from build123d import *

# Parameters (mm, degrees)
BOSS_EXTRUDE2_DEPTH = 16
CUT_EXTRUDE2_DEPTH  = 1
SKETCH6_R           = 0.8
CUT_EXTRUDE4_DEPTH  = 20


with BuildPart() as part:
    # Sketch1 → Revolve2 (revolve)
    with BuildSketch(Plane.XY, mode=Mode.PRIVATE) as revolve2_sk:
        with BuildLine():
            Line((8.97393545, 70), (10, 70))
            Line((10, 70), (10, 85))
            Line((10, 85), (5, 85))
            Line((5, 85), (5, 81.038856971))
            Line((5, 81.038856971), (-25, 81.038856971))
            Line((-25, 81.038856971), (-25, 85))
            Line((-25, 85), (-30, 85))
            Line((-30, 85), (-30, 70))
            add(Edge.make_bspline(
                [(-30, 70), (-18.635717154, 58.062094), (-15, 10)],
                knots=[0, 0, 0, 1, 1, 1], degree=2, weights=[1, 2.302666222, 1]))
            Line((-15, 10), (-15, 0))
            Line((-15, 0), (-9.5, 0))
            Line((-9.5, 0), (-9.5, 4.05))
            Line((-9.5, 4.05), (6.5, 4.05))
            Line((6.5, 4.05), (6.5, 14.05))
            Line((6.5, 14.05), (6.49, 14.05))
            ThreePointArc((6.49, 14.05), (1.90087699, 15.95087699), (0, 20.54))
            Line((0, 20.54), (0, 61.684457842))
            ThreePointArc((0, 61.684457842), (2.856751481, 67.601519544), (8.97393545, 70))
        make_face()
    revolve(revolve2_sk.sketch.rotate(Axis((0, 0, 0), (1, 0, 0)), 90), axis=Axis((0, 0, 0), (1, 0, 0)))

    # Sketch2 → Boss-Extrude2 (add)
    with BuildSketch(Plane(origin=(6.5, 0, 0), x_dir=(0, 0, -1), z_dir=(1, 0, 0))):
        with BuildLine():
            Line((0, -3.05), (-2.664582519, -3.05))
            ThreePointArc((-2.664582519, -3.05), (0, -4.05), (2.664582519, -3.05))
            Line((2.664582519, -3.05), (0, -3.05))
        make_face()
    extrude(amount=-BOSS_EXTRUDE2_DEPTH)

    # Sketch5 → Cut-Extrude2 (cut)
    with BuildSketch(Plane(origin=(10, 0, 0), x_dir=(0, 0, -1), z_dir=(1, 0, 0))):
        Polygon((-10.885951739, 80.726758939), (-9.450054303, 80.726758939), (-9.450054303, 74.162656375), (-7.193644046, 74.162656375), (-7.193644046, 72.726758939), (-10.885951739, 72.726758939), align=None)
        Polygon((-6.629541482, 80.726758939), (-5.031785072, 80.726758939), (-3.603900457, 77.919066632), (-2.172810713, 80.726758939), (-0.578259431, 80.726758939), (-2.885951739, 76.191502529), (-2.885951739, 72.726758939), (-4.321849175, 72.726758939), (-4.321849175, 76.191502529), align=None)
        Polygon((0.908920056, 80.726758939), (2.202189287, 80.726758939), (5.831996979, 75.462335862), (5.831996979, 80.726758939), (7.267894415, 80.726758939), (7.267894415, 72.726758939), (5.9650098, 72.726758939), (2.344817492, 77.975156375), (2.344817492, 72.726758939), (0.908920056, 72.726758939), align=None)
        Polygon((8.62526621, 80.726758939), (10.317573902, 80.726758939), (11.989048261, 78.157848683), (13.663727748, 80.726758939), (15.360843133, 80.726758939), (12.836804672, 76.856566632), (15.524304672, 72.726758939), (13.831996979, 72.726758939), (11.989048261, 75.558489709), (10.142894415, 72.726758939), (8.447381595, 72.726758939), (11.142894415, 76.85977176), align=None)
    extrude(amount=-CUT_EXTRUDE2_DEPTH, mode=Mode.SUBTRACT)

    # Sketch6 → Cut-Extrude4 (cut)
    with BuildSketch(Plane(origin=(0, -3.05, 0), x_dir=(1, 0, 0), z_dir=(0, 1, 0))):
        with Locations(Location((3.805975745, 0, 0), (0, 0, 270))):
            Circle(SKETCH6_R)
    extrude(amount=-CUT_EXTRUDE4_DEPTH, mode=Mode.SUBTRACT)


solid = part.part
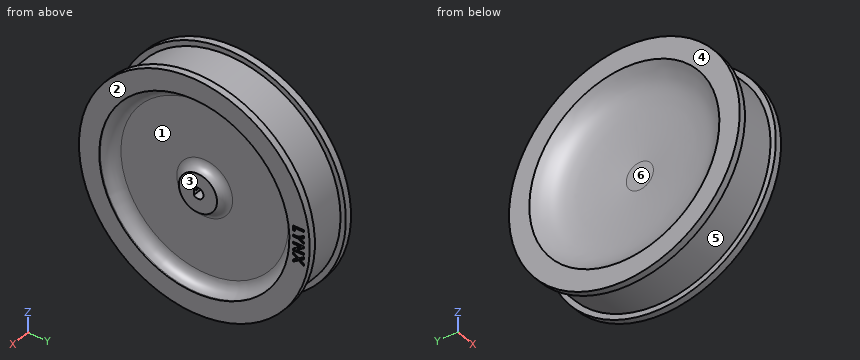
Can you work these out from the model? Positions are in its coordinate system, mm. Face numbers are marked on the shaded views. A direction names the side the tool comes from. Coordinates: 2 decimals unless noted, no trailing zeros. Write each loop counter-clockwise with the first axis right and the second up, starting at its lowest first coordinate (ties: lowest second). Pieces come first, ordered by that corner, then holes. Notation, with made-up numbers: (12.25, 8.25) -> (65.25, 8.25) arc R16 ccw to (65.25, 20.25) -> close; hole circle Ø2 at (66.25, 72.5). An arc over 180 degrees is marked (long way). Write each question's results on one line, items separated by ' | '. Start each with the question number.
Item 1: If we section it at A-A, the plane x = -3.5: Write out the boundary of the cut face in (y, z), and give its area (3 significant figures).
Item 2: I'm going to push flat-ended pins straight in: P1, Ø1.1, axis at x = 9.5, z = -9.5, coming from the +Y side; P2, Ø1.1, axis at x = 9.5, z = -6.5, coming from the +Y side; P3, Ø3, axis at x = -15.5, y = -61.5, coming from the +Z side; P4, Ø1.8, axis at y = 75.5, z = 9.5, coming from the +X side. Where does each tip first touch, or does it pass through?
Item 3: Thinking about a two-plate mould opening in Y: for the marked faces 3, 4, 5 and 6, which applies, released by +Y, released by -Y, zero draft, split by the parting line, or undercut?
Item 4: On a 3-axis mill with a long thin cutter (end or side, diameter ignored), from which of +Z, -Z, +X, -X, +Y, -Y can I reach the whole of each face in a straight line? I mean the marked faces 1 and 2. Say none if no direction works.
Item 5: Please list where these lines run through material, in increasing order: probe 1 along Y at (x, z) = (9.75, 0); probe 2 along Y at (x, z) = (-24, -42); probe 3 along X at (y, z) = (-10.75, 0).
Answer block:
1) outline: circle Ø162.08 at (0, 0); hole (-3.05, -2.66) arc R4.05 ccw (long way) to (-3.05, 2.66) -> close | area: 20,600 mm²
2) P1: y = 84.53 | P2: y = 84.79 | P3: z = 54.47 | P4: x = 10
3) face 3: undercut | face 4: zero draft | face 5: split by the parting line | face 6: undercut
4) face 1: +X | face 2: +Z, -Z, +X, +Y, -Y
5) probe 1: -85 to -70, 70 to 85 | probe 2: -69.31 to -46.46, 46.46 to 69.31 | probe 3: -15.06 to 3.01, 4.61 to 6.5
